```python
from build123d import *

# Parameters (mm, degrees)
F0_W     = 31.5
F0_H     = 19
F0_W_2   = 27.5
F0_H_2   = 15
F1_DEPTH = 20
F0_R     = 2.5
F2_DEPTH = 2.4


with BuildPart() as f1:
    # F0 (on Top) → F1 (new body)
    with BuildSketch(Plane.XY):
        with Locations((13.75, 7.5)):
            Rectangle(F0_W, F0_H)
        with Locations((13.75, 7.5)):
            Rectangle(F0_W_2, F0_H_2, mode=Mode.SUBTRACT)
    extrude(amount=F1_DEPTH)

    # F0 (on Top) → F2 (join)
    with BuildSketch(Plane.XY):
        with Locations((13.75, 7.5)):
            Rectangle(F0_W, F0_H)
        with Locations((13.75, 7.5)):
            Rectangle(F0_W_2, F0_H_2, mode=Mode.SUBTRACT)
        with Locations((13.75, 7.5)):
            Rectangle(F0_W_2, F0_H_2)
        with Locations((13.75, 7.5)):
            Circle(F0_R, mode=Mode.SUBTRACT)
    extrude(amount=-F2_DEPTH)


solid = f1.part
```
Can you work these out from the model? Positions are in its coordinate system, mm. A direction names the side the tool comes from. Coordinates: 2 decimals unless noted, no trailing zeros. Loops run counter-clockwise (first coordinate to the right, second up) from the corner with the lowest first, then second, coordinate; pieces in that order, holes last.
Item 1: Please list where these lines run through material, in increasing order: L1, parallel to Y at x = 13.75, z = -1.05; L2, parallel to X at y = 2.5, z = 11.5; L3, parallel to Y at x = 21.5, z = 19.25.
Answers below:
L1: y = -2 to 5, 10 to 17
L2: x = -2 to 0, 27.5 to 29.5
L3: y = -2 to 0, 15 to 17
Item 2: Suppose I cut it at A-A (z = 4.75). Please give me the cut outline in (x, y), then the cut area to 3 significant figures.
Answers below:
outline: (-2, -2) - (29.5, -2) - (29.5, 17) - (-2, 17) - close; hole (0, 0) - (27.5, 0) - (27.5, 15) - (0, 15) - close
area: 186 mm2
Item 3: If we mould it in two halves opening along Y, with no side actions, what happens to faces 1 (the face through (14, -2, 9)), 2 (the face through (0, 7, 10)), 3 (the face through (10, 8, -2.4))? For each: released by +Y, released by -Y, zero draft, split by the parting line, or undercut.
Answers below:
face 1: released by -Y
face 2: undercut
face 3: zero draft
Item 4: Suppose I cut it at B-B (y = 7.5). Please give me the cut outline in (x, z).
Answers below:
outline: (-2, -2.4) - (11.25, -2.4) - (11.25, 0) - (0, 0) - (0, 20) - (-2, 20) - close; (16.25, -2.4) - (29.5, -2.4) - (29.5, 20) - (27.5, 20) - (27.5, 0) - (16.25, 0) - close
Item 5: Suppose I cut it at C-C (x = 13.75). Please give me the cut outline in (y, z), then the cut area to 3 significant figures.
Answers below:
outline: (-2, -2.4) - (5, -2.4) - (5, 0) - (0, 0) - (0, 20) - (-2, 20) - close; (10, -2.4) - (17, -2.4) - (17, 20) - (15, 20) - (15, 0) - (10, 0) - close
area: 114 mm2
Item 6: Which directions (+Z, -Z, +X, -X, +Y, -Y) give clear straight access to the entire face, cutting with the end or side of a thin tool? Please do faces 4 (the face through (14, 0, 10)), 5 (the face through (14, -1, 20)).
Answers below:
face 4: +Z
face 5: +Z, +X, -X, +Y, -Y
Item 7: Suppose I cut it at D-D (y = 13.5). Please give me the cut outline in (x, z), then the cut area to 3 significant figures.
Answers below:
outline: (-2, -2.4) - (29.5, -2.4) - (29.5, 20) - (27.5, 20) - (27.5, 0) - (0, 0) - (0, 20) - (-2, 20) - close
area: 156 mm2
Item 8: I'm going to push a flat-ended pin straight in: pin 1 (6 mm diameter, centred on x = 13.75, y = 7.5, fed in from +Z). Where does the tip first touch, or does it pass through?
Answers below:
pin 1: stops at z = 0
